Source: CAD feature listing. Evaluate the final solid. Frame: model axes, mm. A direction names the side the tool comes from. Coordinates: 2 decimals unless noted, no trailing zeros. Write each loop counter-clockwise with the first axis right and the second up, starting at its lowest first coordinate (ties: lowest second). Pieces come first, ordered by that corner, then holes. Notation, with made-up numbers: (26.25, 12.25) -> (56.25, 12.25) arc R21 cw to (56.25, 51.25) -> close; hole circle Ø11 at (25, 72). An arc over 180 degrees is marked (long way). One line per item, written item: value. Start each with the question number.
1. Section query D-D, the plane z = -22. Output: boundary loops of the cut face in (x, y), and give its area (3 significant figures).
2. Mould query, pull axis X, two halves, no side actions, for faces 5 (the flat face through (-12.14, 3.45, -11.9)), 6 (the flat face through (-16.442, 3.451, 16.085)), 7 (the flat face through (30, 3, 3.5)). Classes: released by +X, released by -X, zero draft, split by the parting line, or undercut.
3. Access query for faces 1 (the flat face through (3.5, 3, 30)), 2 (the flat face through (-3.5, 3, -30)), 3 (the flat face through (17, 3, -3.5)), 4 (the flat face through (-30, 3, 3.5)). Directions: +Z, -Z, +X, -X, +Y, -Y. A direction counts if a zero-diameter tool reaches every point of the face in a straight line with its end or side. Return the directions, or none.
4. Section query A-A, the plane x = 9.5. Output: boundary loops of the cut face in (y, z).
5. Section query C-C, the plane x = -19. Output: boundary loops of the cut face in (y, z), and give its area (3 significant figures).
6. First-contact query: P1, Ø1, axis at x = -22, y = 1.5, coming from the -Z side; P2, Ø3, axis at x = -30.5, y = 3.5, coming from the +Z side; P3, Ø1, axis at y = 3.5, z = 17.5, coming from the +X side; P4, Ø5, axis at x = -22, z = -14, coming from the -Y side. Flat tips, straight axial feed; report the tip coordinate or a pass-through.
7. Section query B-B, the plane y = 5.75. State how many separate pieces and enclosed holes the cut face has, and give its area (3 significant figures).
8. Line query: line 1 (Z direction, x = 9.5, y = 5.25); line 2 (Z direction, x = -9.5, y = 1.75); line 3 (X direction, y = 3, z = 8). Output: solid intervals per line, ascending.
from build123d import *

# Parameters (mm, degrees)
SKETCH1_R           = 1.5
BOSS_EXTRUDE1_DEPTH = 7


with BuildPart() as part:
    # Sketch1 → Boss-Extrude1 (new body)
    with BuildSketch(Plane(origin=(0, 0, 0), x_dir=(1, 0, 0), z_dir=(0, 1, 0))):
        Polygon((-3.5, -29.026911935), (-3.5, -31.784271247), (3.5, -31.784271247), (3.5, -29.026911935), (29.026911935, -3.5), (31.784271247, -3.5), (31.784271247, 3.5), (29.026911935, 3.5), (3.5, 29.026911935), (3.5, 31.784271247), (-3.5, 31.784271247), (-3.5, 29.026911935), (-29.026911935, 3.5), (-31.784271247, 3.5), (-31.784271247, 0.742640687), (-31.784271247, -3.5), (-29.026911935, -3.5), align=None)
        with BuildLine():
            ThreePointArc((-7.01561146, -19.268659787), (-7.167852395, -20.034026652), (-7.601397898, -20.68287335))
            ThreePointArc((-7.601397898, -20.68287335), (-10.429825023, -20.68287335), (-10.429825023, -17.854446225))
            ThreePointArc((-10.429825023, -17.854446225), (-8.250244595, -17.420900722), (-7.01561146, -19.268659787))
        make_face(mode=Mode.SUBTRACT)
        with BuildLine():
            ThreePointArc((-17.854446225, -10.429825023), (-20.68287335, -10.429825023), (-20.68287335, -7.601397898))
            ThreePointArc((-20.68287335, -7.601397898), (-18.503292923, -7.167852395), (-17.268659787, -9.01561146))
            ThreePointArc((-17.268659787, -9.01561146), (-17.420900722, -9.780978325), (-17.854446225, -10.429825023))
        make_face(mode=Mode.SUBTRACT)
        with BuildLine():
            Line((-3.5, -13.5), (-3.5, -20.54163056))
            Line((-3.5, -20.54163056), (-20.54163056, -3.5))
            Line((-20.54163056, -3.5), (-13.5, -3.5))
            ThreePointArc((-13.5, -3.5), (-6.428932188, -6.428932188), (-3.5, -13.5))
        make_face(mode=Mode.SUBTRACT)
        with Locations((0, -8)):
            Circle(SKETCH1_R, mode=Mode.SUBTRACT)
        with BuildLine():
            ThreePointArc((3.5, -13.5), (6.428932188, -6.428932188), (13.5, -3.5))
            Line((13.5, -3.5), (20.54163056, -3.5))
            Line((20.54163056, -3.5), (3.5, -20.54163056))
            Line((3.5, -20.54163056), (3.5, -13.5))
        make_face(mode=Mode.SUBTRACT)
        with Locations((-9.5, 0)):
            Circle(SKETCH1_R, mode=Mode.SUBTRACT)
        with BuildLine():
            Line((-20.54163056, 3.5), (-3.5, 20.54163056))
            Line((-3.5, 20.54163056), (-3.5, 13.5))
            ThreePointArc((-3.5, 13.5), (-4.261204675, 9.673165676), (-6.428932188, 6.428932188))
            ThreePointArc((-6.428932188, 6.428932188), (-9.673165676, 4.261204675), (-13.5, 3.5))
            Line((-13.5, 3.5), (-20.54163056, 3.5))
        make_face(mode=Mode.SUBTRACT)
        with BuildLine():
            ThreePointArc((3.570714214, 3.5), (4.628907596, 1.890294809), (5, 0))
            ThreePointArc((5, 0), (4.628907596, -1.890294809), (3.570714214, -3.5))
            ThreePointArc((3.570714214, -3.5), (3.535533906, -3.535533906), (3.5, -3.570714214))
            ThreePointArc((3.5, -3.570714214), (0, -5), (-3.5, -3.570714214))
            ThreePointArc((-3.5, -3.570714214), (-3.535533906, -3.535533906), (-3.570714214, -3.5))
            ThreePointArc((-3.570714214, -3.5), (-5, 0), (-3.570714214, 3.5))
            ThreePointArc((-3.570714214, 3.5), (-3.553168481, 3.517810931), (-3.535533906, 3.535533906))
            ThreePointArc((-3.535533906, 3.535533906), (-3.517810931, 3.553168481), (-3.5, 3.570714214))
            ThreePointArc((-3.5, 3.570714214), (-1.890294809, 4.628907596), (0, 5))
            ThreePointArc((0, 5), (1.890294809, 4.628907596), (3.5, 3.570714214))
            ThreePointArc((3.5, 3.570714214), (3.517810931, 3.553168481), (3.535533906, 3.535533906))
            ThreePointArc((3.535533906, 3.535533906), (3.553168481, 3.517810931), (3.570714214, 3.5))
        make_face(mode=Mode.SUBTRACT)
        with BuildLine():
            ThreePointArc((11, 0), (9.5, -1.5), (8, 0))
            ThreePointArc((8, 0), (9.5, 1.5), (11, 0))
        make_face(mode=Mode.SUBTRACT)
        with BuildLine():
            ThreePointArc((0, 6.5), (-1.060660172, 9.060660172), (1.5, 8))
            ThreePointArc((1.5, 8), (1.060660172, 6.939339828), (0, 6.5))
        make_face(mode=Mode.SUBTRACT)
        with BuildLine():
            ThreePointArc((13.5, 3.5), (9.673165676, 4.261204675), (6.428932188, 6.428932188))
            ThreePointArc((6.428932188, 6.428932188), (4.261204675, 9.673165676), (3.5, 13.5))
            Line((3.5, 13.5), (3.5, 20.54163056))
            Line((3.5, 20.54163056), (12.02081528, 12.02081528))
            Line((12.02081528, 12.02081528), (20.54163056, 3.5))
            Line((20.54163056, 3.5), (13.5, 3.5))
        make_face(mode=Mode.SUBTRACT)
        with BuildLine():
            ThreePointArc((20.68287335, 7.601397898), (17.854446225, 7.601397898), (17.854446225, 10.429825023))
            ThreePointArc((17.854446225, 10.429825023), (20.034026652, 10.863370525), (21.268659787, 9.01561146))
            ThreePointArc((21.268659787, 9.01561146), (21.116418852, 8.250244595), (20.68287335, 7.601397898))
        make_face(mode=Mode.SUBTRACT)
        with BuildLine():
            ThreePointArc((10.429825023, 17.854446225), (7.601397898, 17.854446225), (7.601397898, 20.68287335))
            ThreePointArc((7.601397898, 20.68287335), (9.780978325, 21.116418852), (11.01561146, 19.268659787))
            ThreePointArc((11.01561146, 19.268659787), (10.863370525, 18.503292923), (10.429825023, 17.854446225))
        make_face(mode=Mode.SUBTRACT)
    extrude(amount=BOSS_EXTRUDE1_DEPTH)


solid = part.part
Computed values:
1. outline: (-10.53, 0) -> (10.53, 0) -> (10.53, 7) -> (-10.53, 7) -> close
1. area: 147 mm²
2. face 5: undercut
2. face 6: released by -X
2. face 7: zero draft
3. face 1: +Z, +X, +Y, -Y
3. face 2: -Z, -X, +Y, -Y
3. face 3: +Y, -Y
3. face 4: +Z, -X, +Y, -Y
4. outline: (0, -23.03) -> (7, -23.03) -> (7, -21.21) -> (0, -21.21) -> close; (0, -17.33) -> (7, -17.33) -> (7, -14.54) -> (0, -14.54) -> close; (0, -4.33) -> (7, -4.33) -> (7, -1.5) -> (0, -1.5) -> close; (0, 1.5) -> (7, 1.5) -> (7, 4.33) -> (0, 4.33) -> close; (0, 14.54) -> (7, 14.54) -> (7, 23.03) -> (0, 23.03) -> close
5. outline: (0, -13.53) -> (7, -13.53) -> (7, -5.04) -> (0, -5.04) -> close; (0, -3.5) -> (7, -3.5) -> (7, 3.5) -> (0, 3.5) -> close; (0, 5.04) -> (7, 5.04) -> (7, 7.03) -> (0, 7.03) -> close; (0, 11) -> (7, 11) -> (7, 13.53) -> (0, 13.53) -> close
5. area: 140 mm²
6. P1: stops at z = -11.03
6. P2: stops at z = 3.53
6. P3: stops at x = 15.53
6. P4: stops at y = 0
7. separate pieces: 1
7. enclosed holes: 13
7. area: 1,490 mm²
8. line 1: z = -23.03 to -21.21, -17.33 to -14.54, -4.33 to -1.5, 1.5 to 4.33, 14.54 to 23.03
8. line 2: z = -23.03 to -14.54, -4.33 to -1.5, 1.5 to 4.33, 14.54 to 17.33, 21.21 to 23.03
8. line 3: x = -24.53 to -20.99, -17.55 to -16.04, -5.15 to -1.5, 1.5 to 5.15, 16.04 to 24.53
